The listing builds one solid part. Answer for the finished solid, in the listing's coordinates (mm). A direction names the side the tool comes from. Coordinates: 2 decimals unless noted, no trailing zeros. Order: outer loops, then holes, each group sorted by start corner. A loop starts at its lowest first (then second) coordinate and runs counter-clockwise, first axis right, second up. Notation, with made-up numbers: (25.25, 13) -> (53.25, 13) arc R24 cw to (53.25, 32) -> close; hole circle Ø3 at (37.25, 35). An arc over 180 degrees is marked (long way). Put each result on its own line as item: value. Start each with the question number.
```python
from build123d import *

# Parameters (mm, degrees)
BOSS_EXTRUDE1_DEPTH             = 5
SKETCH2_W                       = 300
SKETCH2_H                       = 390
BOSS_EXTRUDE2_DEPTH             = 5
BOSS_EXTRUDE3_DEPTH             = 5
SKETCH4_W                       = 300
SKETCH4_H                       = 254.322327046
BOSS_EXTRUDE4_DEPTH             = 5
SKETCH7_W                       = 300
SKETCH7_H                       = 264.981182322
BOSS_EXTRUDE7_DEPTH             = 5
BOSS_EXTRUDE7_DIRECTION_2_REACH = 597.625


with BuildPart() as part:
    # Sketch1 → Boss-Extrude1 (new body)
    with BuildSketch(Plane(origin=(0, 0, 0), x_dir=(0, 0, -1), z_dir=(1, 0, 0))):
        Polygon((-247.5, 130), (-247.5, -130), (247.5, -130), (141.03222111, 96.195959421), align=None)
    extrude(amount=BOSS_EXTRUDE1_DEPTH)

    # Sketch2 → Boss-Extrude2 (add)
    with BuildSketch(Plane(origin=(0, 107.651495361, -9.366161466), x_dir=(1, 0, 0), z_dir=(0, 0.9962364643840649, -0.08667702712678799))):
        with Locations((-145, -62.836538462)):
            Rectangle(SKETCH2_W, SKETCH2_H)
    extrude(amount=BOSS_EXTRUDE2_DEPTH)

    # Sketch3 → Boss-Extrude3 (add)
    with BuildSketch(Plane.ZY.offset(295)):
        Polygon((247.5, 130), (-141.03222111, 96.195959421), (-247.5, -130), (247.5, -130), align=None)
    extrude(amount=-BOSS_EXTRUDE3_DEPTH)

    # Sketch4 → Boss-Extrude4 (add)
    with BuildSketch(Plane(origin=(0, 71.789415399, -152.520094452), x_dir=(-1, 0, 0), z_dir=(0, 0.42587111556085877, -0.904783837682211))):
        with Locations((145, -95.863836477)):
            Rectangle(SKETCH4_W, SKETCH4_H)
    extrude(amount=BOSS_EXTRUDE4_DEPTH)

    # Sketch7 → Boss-Extrude7 (add)
    with BuildSketch(Plane.XY.offset(247.5)):
        with Locations((-145, 2.490591161)):
            Rectangle(SKETCH7_W, SKETCH7_H)
    extrude(amount=BOSS_EXTRUDE7_DEPTH)

    # Boss-Extrude7 direction 2: up to this face of the body (flat: up to its plane)
    boss_extrude7_direction_2_end = Plane(part.part.faces().sort_by_distance((-145, 132.490591161, 247.283307432))[0])
    # Sketch7 → Boss-Extrude7 direction 2 (add, up to the picked face)
    with BuildSketch(Plane.XY.offset(247.5), mode=Mode.PRIVATE) as boss_extrude7_direction_2_sk1:
        with Locations((-145, 2.490591161)):
            Rectangle(SKETCH7_W, SKETCH7_H)
    boss_extrude7_direction_2_tool1 = split(extrude(boss_extrude7_direction_2_sk1.sketch, amount=-BOSS_EXTRUDE7_DIRECTION_2_REACH, mode=Mode.PRIVATE), bisect_by=boss_extrude7_direction_2_end, keep=Keep.BOTH, mode=Mode.PRIVATE)
    add(boss_extrude7_direction_2_tool1.solids().sort_by(Axis((-145, 2.490591, 247.5), (0, 0, -1)))[0])


solid = part.part
```
(1) A tool of negligible diameter and unlimited length cuts with its end or side. For faces 5 (the flat face through (-147, 4, 252.5)), 6 (the flat face through (-290, 2, 52)), from which of +Z, -Z, +X, -X, +Y, -Y can it reach the whole face along a straight path? Write none if from no direction.
(2) The part is cut by section A-A on y = 84. Determine the outline of the cut face in (x, z).
(3) The part is cut by section B-B on x = -181. Determine the outline of the cut face in (y, z).
(4) The part is cut by section D-D on y = -69.5. Determine the outline of the cut face in (x, z).
(5) Each of these flat-tipped pins is pushed along its axis until it touches: P1, Ø12, axis at x = -180.5, y = 63, coming from the -Z side; P2, Ø3, axis at x = -261, z = -51, coming from the -Y side; P3, Ø1.5, axis at x = -90, z = -122.5, coming from the +Y side. Where does it stop, or does it pass through?
(6) For a pull along X with two mould halves and no side action, classify faces 1 (the flat face through (-142.97, -15.32, -193.52)), 2 (the flat face through (-147.03, 112.86, 50.51)), 3 (the flat face through (-142.9, -11.207, -197.111)), 4 (the flat face through (5, 1, 60)) as released by +X, released by -X, zero draft, split by the parting line, or undercut.
(7) Find the intervals of material crossed by L1, parallel to X at y = 1, z = -72; L2, parallel to Z at x = -14.5, y = 70.5; L3, parallel to Z at x = -22.5, y = 84.5, in increasing order.
(8) The part is cut by section C-C on z = 193.5. Determine the outline of the cut face in (x, y).
Worked out:
1. face 5: +Z, +X, -X, +Y, -Y
1. face 6: -Y
2. outline: (-295, -152.3) -> (5, -152.3) -> (5, 252.5) -> (-295, 252.5) -> close; hole (-290, -146.77) -> (0, -146.77) -> (0, 247.5) -> (-290, 247.5) -> close
3. outline: (-130, -247.5) -> (-127.87, -252.02) -> (102.24, -143.72) -> (101.18, -141.47) -> (134.98, 247.07) -> (134.98, 252.5) -> (-130, 252.5) -> (-130, 247.5) -> (130, 247.5) -> (96.2, -141.03) -> close
4. outline: (-295, -224.55) -> (5, -224.55) -> (5, 252.5) -> (-295, 252.5) -> close; hole (-290, -219.02) -> (0, -219.02) -> (0, 247.5) -> (-290, 247.5) -> close
5. P1: z = -165.01
5. P2: y = 103.9
5. P3: y = 102.89
6. face 1: undercut
6. face 2: undercut
6. face 3: zero draft
6. face 4: released by +X
7. L1: -295 to -290, 0 to 5
7. L2: -158.65 to -153.13, 247.5 to 252.5
7. L3: -152.06 to -146.54, 247.5 to 252.5
8. outline: (-295, -130) -> (-290, -130) -> (-290, 125.3) -> (0, 125.3) -> (0, -130) -> (5, -130) -> (5, 130.32) -> (-295, 130.32) -> close
